```python
from build123d import *

# Parameters (mm, degrees)
SKETCH1_R           = 2.1
BOSS_EXTRUDE1_DEPTH = 729


with BuildPart() as part:
    # Sketch1 → Boss-Extrude1 (new body)
    with BuildSketch(Plane(origin=(0, 0, 0), x_dir=(0, 0, -1), z_dir=(1, 0, 0))):
        with BuildLine():
            Line((10, 13), (10, 19))
            ThreePointArc((10, 19), (9.707106781, 19.707106781), (9, 20))
            Line((9, 20), (3, 20))
            Line((3, 20), (3, 18))
            Line((3, 18), (6, 18))
            Line((6, 18), (6, 17.060660172))
            Line((6, 17.060660172), (2.939339828, 14))
            Line((2.939339828, 14), (-2.939339828, 14))
            Line((-2.939339828, 14), (-6, 17.060660172))
            Line((-6, 17.060660172), (-6, 18))
            Line((-6, 18), (-3, 18))
            Line((-3, 18), (-3, 20))
            Line((-3, 20), (-9, 20))
            ThreePointArc((-9, 20), (-9.707106781, 19.707106781), (-10, 19))
            Line((-10, 19), (-10, -19))
            ThreePointArc((-10, -19), (-9.707106781, -19.707106781), (-9, -20))
            Line((-9, -20), (-3, -20))
            Line((-3, -20), (-3, -18))
            Line((-3, -18), (-6, -18))
            Line((-6, -18), (-6, -17.060660172))
            Line((-6, -17.060660172), (-2.939339828, -14))
            Line((-2.939339828, -14), (2.939339828, -14))
            Line((2.939339828, -14), (6, -17.060660172))
            Line((6, -17.060660172), (6, -18))
            Line((6, -18), (3, -18))
            Line((3, -18), (3, -20))
            Line((3, -20), (9, -20))
            ThreePointArc((9, -20), (9.707106781, -19.707106781), (10, -19))
            Line((10, -19), (10, -13))
            Line((10, -13), (8, -13))
            Line((8, -13), (8, -16))
            Line((8, -16), (7.060660172, -16))
            Line((7.060660172, -16), (4, -12.939339828))
            Line((4, -12.939339828), (4, -7.060660172))
            Line((4, -7.060660172), (7.060660172, -4))
            Line((7.060660172, -4), (8, -4))
            Line((8, -4), (8, -7))
            Line((8, -7), (10, -7))
            Line((10, -7), (10, 7))
            Line((10, 7), (8, 7))
            Line((8, 7), (8, 4))
            Line((8, 4), (7.060660172, 4))
            Line((7.060660172, 4), (4, 7.060660172))
            Line((4, 7.060660172), (4, 12.939339828))
            Line((4, 12.939339828), (7.060660172, 16))
            Line((7.060660172, 16), (8, 16))
            Line((8, 16), (8, 13))
            Line((8, 13), (10, 13))
        make_face()
        with Locations((0, -10)):
            Circle(SKETCH1_R, mode=Mode.SUBTRACT)
        with Locations((0, 10)):
            Circle(SKETCH1_R, mode=Mode.SUBTRACT)
        with BuildLine():
            Line((8, -1.7), (8, 1.7))
            ThreePointArc((8, 1.7), (7.912132034, 1.912132034), (7.7, 2))
            Line((7.7, 2), (7.063603897, 2))
            ThreePointArc((7.063603897, 2), (6.948798867, 2.02283614), (6.851471863, 2.087867966))
            Line((6.851471863, 2.087867966), (2.939339828, 6))
            Line((2.939339828, 6), (-7, 6))
            ThreePointArc((-7, 6), (-7.707106781, 5.707106781), (-8, 5))
            Line((-8, 5), (-8, -5))
            ThreePointArc((-8, -5), (-7.707106781, -5.707106781), (-7, -6))
            Line((-7, -6), (2.939339828, -6))
            Line((2.939339828, -6), (6.851471863, -2.087867966))
            ThreePointArc((6.851471863, -2.087867966), (6.948798867, -2.02283614), (7.063603897, -2))
            Line((7.063603897, -2), (7.7, -2))
            ThreePointArc((7.7, -2), (7.912132034, -1.912132034), (8, -1.7))
        make_face(mode=Mode.SUBTRACT)
        with BuildLine():
            Line((-7.060660172, -16), (-4, -12.939339828))
            Line((-4, -12.939339828), (-4, -8.5))
            ThreePointArc((-4, -8.5), (-4.292893219, -7.792893219), (-5, -7.5))
            Line((-5, -7.5), (-7, -7.5))
            ThreePointArc((-7, -7.5), (-7.707106781, -7.792893219), (-8, -8.5))
            Line((-8, -8.5), (-8, -16))
            Line((-8, -16), (-7.060660172, -16))
        make_face(mode=Mode.SUBTRACT)
        with BuildLine():
            Line((-4, 8.5), (-4, 12.939339828))
            Line((-4, 12.939339828), (-7.060660172, 16))
            Line((-7.060660172, 16), (-8, 16))
            Line((-8, 16), (-8, 8.5))
            ThreePointArc((-8, 8.5), (-7.707106781, 7.792893219), (-7, 7.5))
            Line((-7, 7.5), (-5, 7.5))
            ThreePointArc((-5, 7.5), (-4.292893219, 7.792893219), (-4, 8.5))
        make_face(mode=Mode.SUBTRACT)
    extrude(amount=BOSS_EXTRUDE1_DEPTH)


solid = part.part
```
Can you work these out from the model? Positions are in its coordinate system, mm. Give positions to 0.01 mm unless a question says otherwise; leave off trailing zeros. Use CSV: the item, a comma, the result in double quotes. Start each with the question number.
1. Imagine slicing it at A-A, the plane x = 262. Count the separate pieces of the cut face and the enclosed holes in it, plus the area to 3 significant figures.
2. If I drill on L1, parallel to Y at x = 166.5, z = 0; L2, parallel to Y at x = 426, z = 7.5; L3, parallel to Z at x = 630, y = 11, over which ranges is the centre line in solid material (lowest first)?
3. For P1, Ø1.8, axis at x = 223, z = 0, coming from the -Y side, with a flat end and sliding along its axis, tell me the tip position at first contact or that it passes through.
Response values:
1,separate pieces,"1"
1,enclosed holes,"5"
1,area,"344 mm^2"
2,L1,"-14 to -12.1, -7.9 to -6, 6 to 7.9, 12.1 to 14"
2,L2,"-20 to -16, -7.63 to -5.87, 5.87 to 7.63, 16 to 20"
2,L3,"-4 to -1.85, 1.85 to 4, 8 to 10"
3,P1,"y = -14"
